Design review of the part built by this model. Coordinates are the model's own, in mm. Face numbers are marked on the shaded views. A direction names the side the tool comes from. Round coordinates to 2 decimals unless told otherwise and drop trailing zeros. Order: outer loops, then holes, each group sorted by start corner. A loop starts at its lowest first (then second) coordinate and runs counter-clockwise, first axis right, second up.
from build123d import *

# Parameters (mm, degrees)
F0_W      = 140
F0_H      = 18
F1_DEPTH  = 12
F2_R      = 25
F0_R      = 9
F3_DEPTH  = 24
F0_R_2    = 15
F4_DEPTH  = 24
F5_DEPTH  = 12
F6_DEPTH  = 85
F7_W      = 49
F7_H      = 3
F8_DEPTH  = 140.001
F9_R      = 8
F10_DEPTH = 18.001


with BuildPart() as f1:
    # F0 (on Front) → F1 (new body)
    with BuildSketch(Plane.XZ):
        with BuildLine():
            ThreePointArc((20, 76), (34.142136, 70.142136), (40, 56))
            ThreePointArc((40, 56), (20, 36), (0, 56))
            Line((0, 56), (0, 18))
            Line((0, 18), (140, 18))
            Line((140, 18), (116.866088, 123.870544))
            ThreePointArc((116.866088, 123.870544), (117.341063, 120.952335), (117.5, 118))
            ThreePointArc((117.5, 118), (90, 90.5), (62.5, 118))
            Line((62.5, 118), (62.5, 76))
            Line((62.5, 76), (20, 76))
        make_face()
        with Locations((70, 9)):
            Rectangle(F0_W, F0_H)
    extrude(amount=F1_DEPTH)

    # F2
    f2_edges = [f1.edges().sort_by_distance(p)[0] for p in [
        (62.5, -6, 76),
    ]]
    fillet(f2_edges, radius=F2_R)

    # F0 (on Front) → F3 (join)
    with BuildSketch(Plane.XZ):
        with BuildLine():
            ThreePointArc((0, 56), (20, 36), (40, 56))
            ThreePointArc((40, 56), (34.142136, 70.142136), (20, 76))
            ThreePointArc((20, 76), (5.857864, 70.142136), (0, 56))
        make_face()
        with Locations((20, 56)):
            Circle(F0_R, mode=Mode.SUBTRACT)
    extrude(amount=F3_DEPTH)

    # F0 (on Front) → F4 (join)
    with BuildSketch(Plane.XZ):
        with BuildLine():
            ThreePointArc((116.866088, 123.870544), (87.047665, 145.341063), (62.5, 118))
            ThreePointArc((62.5, 118), (90, 90.5), (117.5, 118))
            ThreePointArc((117.5, 118), (117.341063, 120.952335), (116.866088, 123.870544))
        make_face()
        with Locations((90, 118)):
            Circle(F0_R_2, mode=Mode.SUBTRACT)
    extrude(amount=F4_DEPTH)

    # F0 (on Front) → F5 (join)
    with BuildSketch(Plane.XZ):
        with BuildLine():
            ThreePointArc((116.866088, 123.870544), (87.047665, 145.341063), (62.5, 118))
            ThreePointArc((62.5, 118), (90, 90.5), (117.5, 118))
            ThreePointArc((117.5, 118), (117.341063, 120.952335), (116.866088, 123.870544))
        make_face()
        with Locations((90, 118)):
            Circle(F0_R_2, mode=Mode.SUBTRACT)
    extrude(amount=-F5_DEPTH)

    # F0 (on Front) → F6 (join)
    with BuildSketch(Plane.XZ):
        with Locations((70, 9)):
            Rectangle(F0_W, F0_H)
    extrude(amount=F6_DEPTH)

    # F7 (on face) → F8 (cut, through all)
    with BuildSketch(Plane(origin=(0, 0, 0), x_dir=(0, -1, 0), z_dir=(-1, 0, 0))):
        with Locations((42.5, 1.5)):
            Rectangle(F7_W, F7_H)
    extrude(amount=-F8_DEPTH, mode=Mode.SUBTRACT)

    # F9 (on face) → F10 (cut, through all)
    with BuildSketch(Plane.XY.offset(18)):
        with Locations((35, -55)):
            Circle(F9_R)
        with Locations((105, -55)):
            Circle(F9_R)
    extrude(amount=-F10_DEPTH, mode=Mode.SUBTRACT)


solid = f1.part
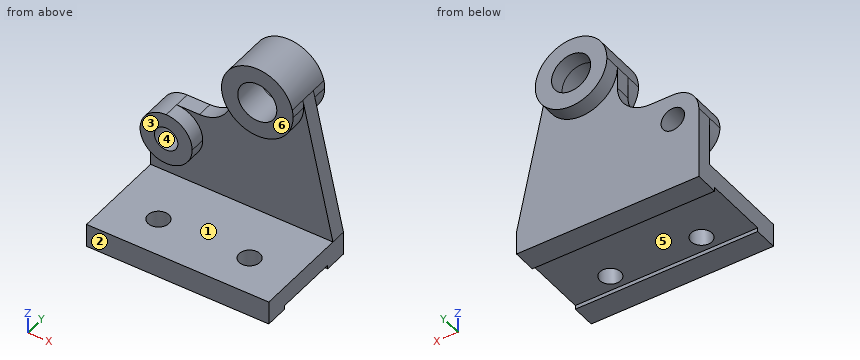
1) Clearance check with flat-ended pins moving along their axes: P1, Ø1.5, axis at x = 95, z = 77, coming from the +Y side; P2, Ø5, axis at x = 121.5, z = 67, coming from the -Y side; P3, Ø1.5, axis at x = 68.5, z = 124.5, coming from the -Y side. State where each tip first meets the part, or that it passes through.
Results:
P1: stops at y = 0
P2: stops at y = -12
P3: stops at y = -24
2) Take a section at D-D on z = 60. Give the boundary of the cut face in (x, y), plus the area to 3 significant figures.
Results:
outline: (0.4, -24) - (11.94, -24) - (11.94, 0) - (0.4, 0) - close; (28.06, -24) - (39.6, -24) - (39.6, -12) - (130.82, -12) - (130.82, 0) - (28.06, 0) - close
area: 1,650 mm2
3) The part is to be moulded in two halves that separate along Z. For the marked faces 4, 5 and 6, say which applies: released by +Z, released by -Z, zero draft, split by the parting line, or undercut.
Results:
face 4: undercut
face 5: released by -Z
face 6: zero draft
4) Take a section at C-C on y = -55. Give the boundary of the cut face in (x, z).
Results:
outline: (0, 3) - (27, 3) - (27, 18) - (0, 18) - close; (43, 3) - (97, 3) - (97, 18) - (43, 18) - close; (113, 3) - (140, 3) - (140, 18) - (113, 18) - close
5) Take a section at A-A on y = -21.5. Give the boundary of the cut face in (x, z).
Results:
outline: (0, 3) - (140, 3) - (140, 18) - (0, 18) - close; (0, 56) arc R20 ccw to (40, 56) arc R20 ccw to (20, 76) arc R20 ccw to start; (116.87, 123.87) arc R27.5 ccw (long way) to (117.5, 118) arc R27.5 ccw to start; hole circle Ø18 at (20, 56); hole circle Ø30 at (90, 118)
6) Take a section at B-B on x = 90. Give the boundary of the cut face in (y, z), plus the area to 3 significant figures.
Results:
outline: (-85, 0) - (-67, 0) - (-67, 3) - (-18, 3) - (-18, 0) - (0, 0) - (0, 90.5) - (12, 90.5) - (12, 103) - (-24, 103) - (-24, 90.5) - (-12, 90.5) - (-12, 18) - (-85, 18) - close; (-24, 133) - (12, 133) - (12, 145.5) - (-24, 145.5) - close
area: 3,150 mm2
7) For the marked faces 1, 2 and 3, list the 3-axis set-ups (+Z, -Z, +X, -X, +Y, -Y) from which the entire face can be reached by the end or side of a thin tool; tool diameter is ignored.
Results:
face 1: +X, -X, -Y
face 2: +Z, -Z, +X, -X, -Y
face 3: +Z, +X, -X, -Y
8) To check wall thickness, follow line 1 along Z through (x, y) = (90, -15.25); line 2 along Y through (x, z) = (35, 13.25); line 3 along Z through (x, y) = (59, -76.5). State the ranges of each line that lie inside material, in increasing order.
Results:
line 1: z = 0 to 18, 90.5 to 103, 133 to 145.5
line 2: y = -85 to -63, -47 to 0
line 3: z = 0 to 18
